The model under review builds one solid part; all positions refer to its coordinate system, in mm. Face numbers are marked on the shaded views. A direction names the side the tool comes from. Give positions to 0.01 mm unless a question says otherwise; leave off trailing zeros. Loops run counter-clockwise (first coordinate to the right, second up) from the corner with the lowest first, then second, coordinate; pieces in that order, holes last. Notation, with made-up numbers: (-36.5, 10) - (-28.5, 10) arc R31 ccw to (-28.5, 37) - close; hole circle Ø9 at (23, 10.25). An arc over 180 degrees is marked (long way). Answer as a JSON object with one key per item and string values.
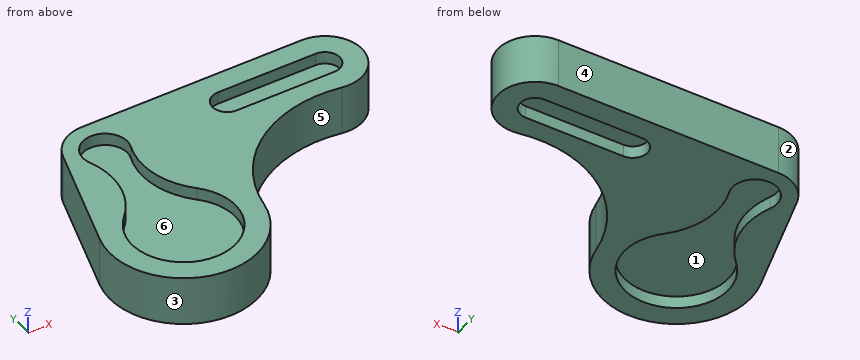
from build123d import *

# Parameters (mm, degrees)
BOSS_EXTRUDE1_DEPTH   = 5
BOSS_EXTRUDE1_2_DEPTH = 5
BOSS_EXTRUDE2_START   = -10
BOSS_EXTRUDE2_DEPTH   = 20


with BuildPart() as part:
    # Sketch1 → Boss-Extrude1 (new, symmetric)
    with BuildSketch(Plane.XY):
        with BuildLine():
            Line((90, 44), (50, 44))
            ThreePointArc((50, 44), (44, 50), (50, 56))
            Line((50, 56), (90, 56))
            ThreePointArc((90, 56), (96, 50), (90, 44))
        make_face()
    extrude(amount=BOSS_EXTRUDE1_DEPTH, both=True)



with BuildPart() as body_2:
    # Sketch1 → Boss-Extrude1 2 (new, symmetric)
    with BuildSketch(Plane.XY):
        with BuildLine():
            ThreePointArc((-14.956527547, 14.741176471), (0, -21), (14.956527547, 14.741176471))
            ThreePointArc((14.956527547, 14.741176471), (6.937432482, 29.759413292), (8.382229724, 46.723076923))
            ThreePointArc((8.382229724, 46.723076923), (0, 59), (-8.382229724, 46.723076923))
            ThreePointArc((-8.382229724, 46.723076923), (-6.937432482, 29.759413292), (-14.956527547, 14.741176471))
        make_face()
    extrude(amount=BOSS_EXTRUDE1_2_DEPTH, both=True)


with BuildPart() as part_1:
    add(part.part)

    add(body_2.part)  # Boss-Extrude2 merges body 2
    # Sketch1<4> → Boss-Extrude2 (add)
    with BuildSketch(Plane.XY.offset(BOSS_EXTRUDE2_START)):
        with BuildLine():
            Line((0, 65), (90, 65))
            ThreePointArc((90, 65), (104.943418217, 48.698365648), (87.406551135, 35.225900265))
            ThreePointArc((87.406551135, 35.225900265), (50.100874494, 26.949083525), (29.535645594, -5.25791207))
            ThreePointArc((29.535645594, -5.25791207), (-7.143700144, -29.137047693), (-28.618176043, 9))
            Line((-28.618176043, 9), (-14.309088021, 54.5))
            ThreePointArc((-14.309088021, 54.5), (-8.874119675, 62.093386622), (0, 65))
        make_face()
        with BuildLine():
            Line((90, 44), (50, 44))
            ThreePointArc((50, 44), (44, 50), (50, 56))
            Line((50, 56), (90, 56))
            ThreePointArc((90, 56), (96, 50), (90, 44))
        make_face(mode=Mode.SUBTRACT)
        with BuildLine():
            ThreePointArc((-14.956527547, 14.741176471), (0, -21), (14.956527547, 14.741176471))
            ThreePointArc((14.956527547, 14.741176471), (6.937432482, 29.759413292), (8.382229724, 46.723076923))
            ThreePointArc((8.382229724, 46.723076923), (0, 59), (-8.382229724, 46.723076923))
            ThreePointArc((-8.382229724, 46.723076923), (-6.937432482, 29.759413292), (-14.956527547, 14.741176471))
        make_face(mode=Mode.SUBTRACT)
    extrude(amount=BOSS_EXTRUDE2_DEPTH)


solid = part_1.part
Q1. Consider section C-C, the plane z = 2. State the section outline as (x, y) points.
Results:
{"outline": "(-28.62, 9) arc R30 ccw (long way) to (29.54, -5.26) arc R50 cw to (87.41, 35.23) arc R15 ccw (long way) to (90, 65) - (0, 65) arc R15 ccw to (-14.31, 54.5) - close"}
Q2. Consider section A-A, the plane y = 7. State the section outline as (x, z) points, plus the area to 3 significant figures.
Results:
{"outline": "(-29.17, -10) - (-19.8, -10) - (-19.8, -5) - (19.8, -5) - (19.8, -10) - (33.4, -10) - (33.4, 10) - (19.8, 10) - (19.8, 5) - (-19.8, 5) - (-19.8, 10) - (-29.17, 10) - close", "area": "855 mm^2"}
Q3. Consider section D-D, the plane y = 50. State the section outline as (x, z) points.
Results:
{"outline": "(-15.72, -10) - (-9, -10) - (-9, -5) - (9, -5) - (9, -10) - (44, -10) - (44, -5) - (96, -5) - (96, -10) - (105, -10) - (105, 10) - (96, 10) - (96, 5) - (44, 5) - (44, 10) - (9, 10) - (9, 5) - (-9, 5) - (-9, 10) - (-15.72, 10) - close"}
Q4. Clearance check with flat-ended pins moving along their axes: pin 1 Ø12 at (y, z) = (48, 3) entering from -X; pin 2 Ø3 at (x, y) = (-2.5, 3) entering from -Z; pin 3 Ø2 at (x, y) = (67.5, 49) entering from +Z. State where each tip first meets the part, or that it passes through.
Results:
{"pin 1": "stops at x = -18.24", "pin 2": "stops at z = -5", "pin 3": "stops at z = 5"}
Q5. The part is to be moulded in two halves that separate along X. For the marked faces 1, 2, 3 and 4, say which applies: +X half, -X half, draft (parallel to the pull), parting line (faces both ways), or undercut.
Results:
{"face 1": "undercut", "face 2": "-X half", "face 3": "parting line", "face 4": "draft"}
Q6. Consider section B-B, the plane x = 67. State the section outline as (y, z) points.
Results:
{"outline": "(34.58, -10) - (44, -10) - (44, -5) - (56, -5) - (56, -10) - (65, -10) - (65, 10) - (56, 10) - (56, 5) - (44, 5) - (44, 10) - (34.58, 10) - close"}
Q7. For the marked faces 5 and 6, list the 3-axis set-ups (+Z, -Z, +X, -X, +Y, -Y) from which the entire face can be reached by the end or side of a thin tool; tool diameter is ignored.
Results:
{"face 5": "+Z, -Z, -Y", "face 6": "+Z"}
Q8. To check wall thickness, follow probe 1 along X at (y, z) = (50, -6.9); probe 2 along Z at (x, y) = (-2.5, 8); probe 3 along X at (y, z) = (0, 7.05). State the ranges of each line that lie inside material, in increasing order. Write a range as [from, to].
Results:
{"probe 1": "x = [-15.72, -9], [9, 44], [96, 105]", "probe 2": "z = [-5, 5]", "probe 3": "x = [-30, -21], [21, 30.77]"}
